Could you check a few things on this drawing? It's one solid part, dimensions in mm from its lowest x, y, z. A direction names the side the tool comes from. Give positions to 0.01 mm unless a question says otherwise; leave off trailing zeros. Loops run counter-clockwise (first coordinate to the right, second up) from the corner with the lowest first, then second, coordinate; pieces in that order, holes last. Notation, with made-up numbers: (87, 73) - (104, 73) arc R16 cw to (104, 103) - close; hole circle Ø7 at (-3, 56). An arc over 180 degrees is marked (long way). Return JSON: item names as keys, results as strings. Group by question number.
(1) I need wall thicknesses on probe 1 along Y at (x, z) = (6.75, 23); probe 2 along Z at (x, y) = (4.5, 4.25); probe 3 along Z at (x, y) = (2, 6.75). Which ranges of each line are inside material? Lowest first, please. Write a range as [from, to].
(2) If we section it at D-D (z = 5.5): Please give me the cut outline in (x, y), then the cut area to 3 significant figures.
(3) If we section it at A-A (x = 3.5): Please give me the cut outline in (y, z).
(4) For P1, Ø3, axis at x = 2, z = 13.5, coming from the -Y side, with a flat end and sliding along its axis, tell me the tip position at first contact or that it passes through.
(5) If we section it at B-B (z = 31.5): Please give me the cut outline in (x, y), then the cut area to 3 significant figures.
(6) If we section it at C-C (y = 11.5): Please give me the cut outline in (x, z).
(7) On a 3-axis mill with a long thin cutter (end or side, diameter ignored), from which of +Z, -Z, +X, -X, +Y, -Y can I reach the whole of each face in a straight line? I mean the marked faces 1 and 2. Say none if no direction works.
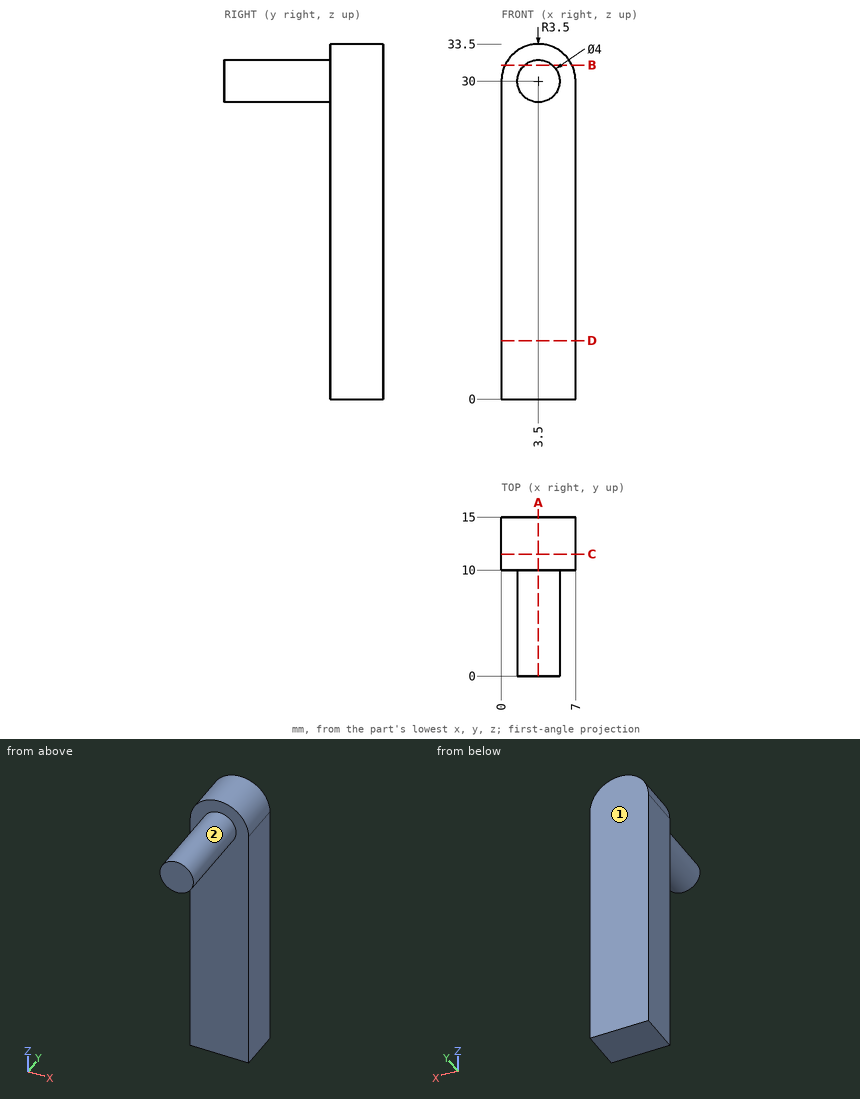
Values:
{
 "1": {"probe 1": "[10, 15]", "probe 2": "[28.27, 31.73]", "probe 3": "[28.68, 31.32]"},
 "2": {"outline": "(0, 10) - (7, 10) - (7, 15) - (0, 15) - close", "area": "35.0 mm2"},
 "3": {"outline": "(0, 28) - (10, 28) - (10, 0) - (15, 0) - (15, 33.5) - (10, 33.5) - (10, 32) - (0, 32) - close"},
 "4": {"P1": "y = 10"},
 "5": {"outline": "(0.34, 10) - (2.18, 10) - (2.18, 0) - (4.82, 0) - (4.82, 10) - (6.66, 10) - (6.66, 15) - (0.34, 15) - close", "area": "58.1 mm2"},
 "6": {"outline": "(0, 0) - (7, 0) - (7, 30) arc R3.5 ccw to (0, 30) - close"},
 "7": {"face 1": "+Z, -Z, +X, -X, +Y", "face 2": "-Y"}
}
